Design review of the part built by this model. Coordinates are the model's own, in mm. Face numbers are marked on the shaded views. Round coordinates to 2 decimals unless told otherwise and drop trailing zeros. Order: outer loops, then holes, each group sorted by start corner. A loop starts at its lowest first (then second) coordinate and runs counter-clockwise, first axis right, second up.
from build123d import *

# Parameters (mm, degrees)
BOSS_EXTRUDE1_DEPTH = 31.75
SKETCH2_R           = 1.6383
SKETCH2_W           = 6.35
SKETCH2_H           = 4.826
CUT_EXTRUDE1_DEPTH  = 4.175
BOSS_EXTRUDE2_REACH = 21.05
SKETCH3_R           = 0.9525


with BuildPart() as part:
    # Sketch1 → Boss-Extrude1 (new body)
    with BuildSketch(Plane.XY):
        with BuildLine():
            Line((1.5875, 0), (1.5875, -9.5885))
            Line((1.5875, -9.5885), (1.0287, -9.5885))
            Line((1.0287, -9.5885), (1.0287, -1.209104032))
            ThreePointArc((1.0287, -1.209104032), (0, -1.5875), (-1.0287, -1.209104032))
            Line((-1.0287, -1.209104032), (-1.0287, -9.5885))
            Line((-1.0287, -9.5885), (-1.5875, -9.5885))
            Line((-1.5875, -9.5885), (-1.5875, 0))
            ThreePointArc((-1.5875, 0), (0, 1.5875), (1.5875, 0))
        make_face()
    extrude(amount=BOSS_EXTRUDE1_DEPTH)

    # Sketch2 → Cut-Extrude1 (cut, through all)
    with BuildSketch(Plane(origin=(1.5875, 0, 0), x_dir=(0, 0, -1), z_dir=(1, 0, 0))):
        with Locations((-28.575, -6.0071)):
            Circle(SKETCH2_R)
        with Locations((-3.175, -6.0071)):
            Circle(SKETCH2_R)
        with Locations((-15.875, -0.8255)):
            Rectangle(SKETCH2_W, SKETCH2_H)
    extrude(amount=-CUT_EXTRUDE1_DEPTH, mode=Mode.SUBTRACT)

    # Sketch3 → Boss-Extrude2 (add, up to next)
    with BuildSketch(Plane.XY.offset(12.7), mode=Mode.PRIVATE) as boss_extrude2_sk1:
        Circle(SKETCH3_R)
    boss_extrude2_tool1 = extrude(boss_extrude2_sk1.sketch, amount=BOSS_EXTRUDE2_REACH, mode=Mode.PRIVATE) - part.part
    add(boss_extrude2_tool1.solids().sort_by_distance((0, 0, 12.7))[0])


solid = part.part
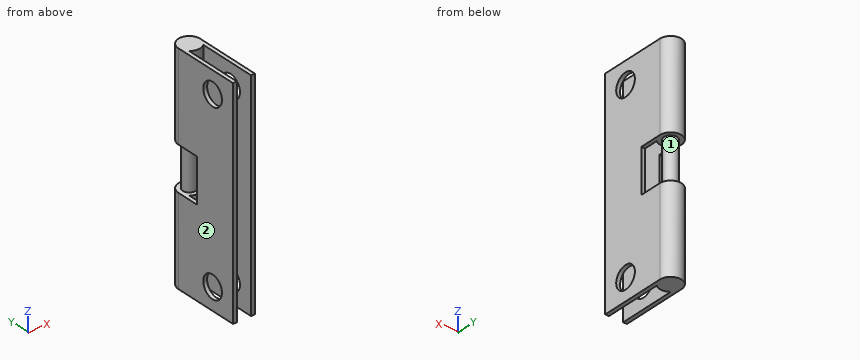
1) Take a section at A-A on z = 18. Give the boundary of the cut face in (x, y) (1 decimal), plus the area to 3 significant figures.
Results:
outline: (-1.6, -9.6) - (-1, -9.6) - (-1, -3.2) - (-1.6, -3.2) - close; circle Ø1.9 at (0, 0); (1, -9.6) - (1.6, -9.6) - (1.6, -3.2) - (1, -3.2) - close
area: 9.95 mm2
2) Take a section at C-C on x = 0. Give the boundary of the cut face in (y, z).
Results:
outline: (-1.59, 0) - (1.59, 0) - (1.59, 12.7) - (0.95, 12.7) - (0.95, 19.05) - (1.59, 19.05) - (1.59, 31.75) - (-1.59, 31.75) - (-1.59, 19.05) - (-0.95, 19.05) - (-0.95, 12.7) - (-1.59, 12.7) - close
3) Take a section at B-B on y = -2. Give the boundary of the cut face in (x, z), plus the area to 3 significant figures.
Results:
outline: (-1.59, 0) - (-1.03, 0) - (-1.03, 12.7) - (-1.59, 12.7) - close; (-1.59, 19.05) - (-1.03, 19.05) - (-1.03, 31.75) - (-1.59, 31.75) - close; (1.03, 0) - (1.59, 0) - (1.59, 12.7) - (1.03, 12.7) - close; (1.03, 19.05) - (1.59, 19.05) - (1.59, 31.75) - (1.03, 31.75) - close
area: 28.4 mm2
4) Take a section at D-D on y = -3.75. Give the boundary of the cut face in (x, z), plus the area to 3 significant figures.
Results:
outline: (-1.59, 0) - (-1.03, 0) - (-1.03, 31.75) - (-1.59, 31.75) - close; (1.03, 0) - (1.59, 0) - (1.59, 31.75) - (1.03, 31.75) - close
area: 35.5 mm2
5) The part is to be moulded in two halves that separate along Z. For the marked faces 1 and 2, say which applies: released by +Z, released by -Z, zero draft, split by the parting line, or undercut.
Results:
face 1: undercut
face 2: zero draft
6) Clearance check with a flat-ended pin moving along its axis: P1, Ø0.6, axis at x = 1.5, z = 15, coming from the +Y side. State where the tip first meets the part, or that it passes through.
Results:
P1: stops at y = -3.24
7) To check wall thickness, follow line 1 along Z through (x, y) = (-0.95, -0.5); line 2 along X through (y, z) = (-5, 14.5); line 3 along Y through (x, z) = (0.1, 2.5). State the ranges of each line that lie inside material, in increasing order.
Results:
line 1: z = 0 to 12.7, 19.05 to 31.75
line 2: x = -1.59 to -1.03, 1.03 to 1.59
line 3: y = -1.58 to 1.58
